Could you check a few things on this model? Use its own coordinates, in mm. A direction names the side the tool comes from. Give positions to 0.01 mm unless a question says otherwise; leave off trailing zeros. Write each loop counter-clockwise with the first axis right and the second up, starting at its lowest first coordinate (ties: lowest second). Pieces come first, ordered by that corner, then holes. Notation, with made-up numbers: M -23,46.5 L 18,46.5 A10 cw 18,62.5 Z; hole C -26,80.5 d2. An arc over 180 degrees is marked long. One line per item, written item: value.
```python
from build123d import *

# Parameters (mm, degrees)
SKETCH1_W           = 119.5324
SKETCH1_H           = 78.0034
BOSS_EXTRUDE1_DEPTH = 1.5875
CUT_EXTRUDE1_REACH  = 3.587
SKETCH2_R           = 2
SKETCH3_R           = 0.508
CUT_EXTRUDE2_DEPTH  = 1.5875
CUT_EXTRUDE4_REACH  = 3.587
LPATTERN1_COUNT     = 26
LPATTERN1_PITCH     = 2.54
SKETCH5_W           = 105.5
SKETCH5_H           = 67.2
BOSS_EXTRUDE2_DEPTH = 5.08
SKETCH6_W           = 98.5
SKETCH6_H           = 57.4
CUT_EXTRUDE3_DEPTH  = 0.127
SKETCH7_W           = 6
SKETCH7_H           = 3.5
BOSS_EXTRUDE3_DEPTH = 3.8
SKETCH8_W           = 3
SKETCH8_H           = 1.5
BOSS_EXTRUDE4_DEPTH = 0.7
SKETCH9_W           = 3
SKETCH9_H           = 3
BOSS_EXTRUDE5_DEPTH = 1.71
SKETCH10_W          = 3
SKETCH10_H          = 3
BOSS_EXTRUDE6_DEPTH = 1


with BuildPart() as part:
    # Sketch1 → Boss-Extrude1 (new body)
    with BuildSketch(Plane(origin=(0, 0, 0), x_dir=(1, 0, 0), z_dir=(0, 1, 0))):
        Rectangle(SKETCH1_W, SKETCH1_H)
    extrude(amount=BOSS_EXTRUDE1_DEPTH)

    # Sketch2 → Cut-Extrude1 (cut, up to next)
    with BuildSketch(Plane(origin=(0, 1.5875, 0), x_dir=(1, 0, 0), z_dir=(0, 1, 0)), mode=Mode.PRIVATE) as cut_extrude1_sk1:
        with Locations((-55.7657, 35.0012)):
            Circle(SKETCH2_R)
    cut_extrude1_tool1 = extrude(cut_extrude1_sk1.sketch, amount=-CUT_EXTRUDE1_REACH, mode=Mode.PRIVATE) & part.part
    add(cut_extrude1_tool1.solids().sort_by_distance((-55.7657, 1.5875, -35.0012))[0], mode=Mode.SUBTRACT)
    # Sketch2 → Cut-Extrude1 (cut, up to next)
    with BuildSketch(Plane(origin=(0, 1.5875, 0), x_dir=(1, 0, 0), z_dir=(0, 1, 0)), mode=Mode.PRIVATE) as cut_extrude1_sk2:
        with Locations((-55.7657, -35.0012)):
            Circle(SKETCH2_R)
    cut_extrude1_tool2 = extrude(cut_extrude1_sk2.sketch, amount=-CUT_EXTRUDE1_REACH, mode=Mode.PRIVATE) & part.part
    add(cut_extrude1_tool2.solids().sort_by_distance((-55.7657, 1.5875, 35.0012))[0], mode=Mode.SUBTRACT)
    # Sketch2 → Cut-Extrude1 (cut, up to next)
    with BuildSketch(Plane(origin=(0, 1.5875, 0), x_dir=(1, 0, 0), z_dir=(0, 1, 0)), mode=Mode.PRIVATE) as cut_extrude1_sk3:
        with Locations((55.7657, 35.0012)):
            Circle(SKETCH2_R)
    cut_extrude1_tool3 = extrude(cut_extrude1_sk3.sketch, amount=-CUT_EXTRUDE1_REACH, mode=Mode.PRIVATE) & part.part
    add(cut_extrude1_tool3.solids().sort_by_distance((55.7657, 1.5875, -35.0012))[0], mode=Mode.SUBTRACT)
    # Sketch2 → Cut-Extrude1 (cut, up to next)
    with BuildSketch(Plane(origin=(0, 1.5875, 0), x_dir=(1, 0, 0), z_dir=(0, 1, 0)), mode=Mode.PRIVATE) as cut_extrude1_sk4:
        with Locations((55.7657, -35.0012)):
            Circle(SKETCH2_R)
    cut_extrude1_tool4 = extrude(cut_extrude1_sk4.sketch, amount=-CUT_EXTRUDE1_REACH, mode=Mode.PRIVATE) & part.part
    add(cut_extrude1_tool4.solids().sort_by_distance((55.7657, 1.5875, 35.0012))[0], mode=Mode.SUBTRACT)

    # Sketch3 → Cut-Extrude2 (cut)
    with BuildSketch(Plane(origin=(0, 1.5875, 0), x_dir=(1, 0, 0), z_dir=(0, 1, 0))):
        with Locations((-31.7373, 36.758)):
            Circle(SKETCH3_R)
        with Locations((-31.7373, -36.758)):
            Circle(SKETCH3_R)
    cut_extrude2 = extrude(amount=-CUT_EXTRUDE2_DEPTH, mode=Mode.SUBTRACT)

    # Sketch11 → Cut-Extrude4 (cut, up to next)
    with BuildSketch(Plane(origin=(0, 1.5875, 0), x_dir=(1, 0, 0), z_dir=(0, 1, 0)), mode=Mode.PRIVATE) as cut_extrude4_sk1:
        with BuildLine():
            Line((-59.7662, 35.0012), (-59.7662, 39.0017))
            Line((-59.7662, 39.0017), (-55.7657, 39.0017))
            ThreePointArc((-55.7657, 39.0017), (-58.594480678, 37.829980678), (-59.7662, 35.0012))
        make_face()
    cut_extrude4_tool1 = extrude(cut_extrude4_sk1.sketch, amount=-CUT_EXTRUDE4_REACH, mode=Mode.PRIVATE) & part.part
    add(cut_extrude4_tool1.solids().sort_by_distance((-58.872617, 1.5875, -38.108117))[0], mode=Mode.SUBTRACT)
    # Sketch11 → Cut-Extrude4 (cut, up to next)
    with BuildSketch(Plane(origin=(0, 1.5875, 0), x_dir=(1, 0, 0), z_dir=(0, 1, 0)), mode=Mode.PRIVATE) as cut_extrude4_sk2:
        with BuildLine():
            Line((-59.7662, -39.0017), (-55.7657, -39.0017))
            ThreePointArc((-55.7657, -39.0017), (-58.594480678, -37.829980678), (-59.7662, -35.0012))
            Line((-59.7662, -35.0012), (-59.7662, -39.0017))
        make_face()
    cut_extrude4_tool2 = extrude(cut_extrude4_sk2.sketch, amount=-CUT_EXTRUDE4_REACH, mode=Mode.PRIVATE) & part.part
    add(cut_extrude4_tool2.solids().sort_by_distance((-58.872617, 1.5875, 38.108117))[0], mode=Mode.SUBTRACT)
    # Sketch11 → Cut-Extrude4 (cut, up to next)
    with BuildSketch(Plane(origin=(0, 1.5875, 0), x_dir=(1, 0, 0), z_dir=(0, 1, 0)), mode=Mode.PRIVATE) as cut_extrude4_sk3:
        with BuildLine():
            Line((59.7662, -35.0012), (59.7662, -39.0017))
            Line((59.7662, -39.0017), (55.7657, -39.0017))
            ThreePointArc((55.7657, -39.0017), (58.594480678, -37.829980678), (59.7662, -35.0012))
        make_face()
    cut_extrude4_tool3 = extrude(cut_extrude4_sk3.sketch, amount=-CUT_EXTRUDE4_REACH, mode=Mode.PRIVATE) & part.part
    add(cut_extrude4_tool3.solids().sort_by_distance((58.872617, 1.5875, 38.108117))[0], mode=Mode.SUBTRACT)
    # Sketch11 → Cut-Extrude4 (cut, up to next)
    with BuildSketch(Plane(origin=(0, 1.5875, 0), x_dir=(1, 0, 0), z_dir=(0, 1, 0)), mode=Mode.PRIVATE) as cut_extrude4_sk4:
        with BuildLine():
            Line((59.7662, 39.0017), (55.7657, 39.0017))
            ThreePointArc((55.7657, 39.0017), (58.594480678, 37.829980678), (59.7662, 35.0012))
            Line((59.7662, 35.0012), (59.7662, 39.0017))
        make_face()
    cut_extrude4_tool4 = extrude(cut_extrude4_sk4.sketch, amount=-CUT_EXTRUDE4_REACH, mode=Mode.PRIVATE) & part.part
    add(cut_extrude4_tool4.solids().sort_by_distance((58.872617, 1.5875, -38.108117))[0], mode=Mode.SUBTRACT)

    # LPattern1: Cut-Extrude2 ×26
    with Locations(*[(i * LPATTERN1_PITCH, 0, 0) for i in range(1, LPATTERN1_COUNT)]):
        add(cut_extrude2, mode=Mode.SUBTRACT)

    # Sketch5 → Boss-Extrude2 (add)
    with BuildSketch(Plane(origin=(0, 1.5875, 0), x_dir=(1, 0, 0), z_dir=(0, 1, 0))):
        with Locations((0.0838, 0.4017)):
            Rectangle(SKETCH5_W, SKETCH5_H)
    extrude(amount=BOSS_EXTRUDE2_DEPTH)

    # Sketch6 → Cut-Extrude3 (cut)
    with BuildSketch(Plane(origin=(0, 6.6675, 0), x_dir=(1, 0, 0), z_dir=(0, 1, 0))):
        with Locations((0.0838, 2.8017)):
            Rectangle(SKETCH6_W, SKETCH6_H)
    extrude(amount=-CUT_EXTRUDE3_DEPTH, mode=Mode.SUBTRACT)

    # Sketch7 → Boss-Extrude3 (add)
    with BuildSketch(Plane(origin=(0, 1.5875, 0), x_dir=(1, 0, 0), z_dir=(0, 1, 0))):
        with Locations((-42.2662, 36.2517)):
            Rectangle(SKETCH7_W, SKETCH7_H)
    extrude(amount=BOSS_EXTRUDE3_DEPTH)

    # Sketch8 → Boss-Extrude4 (add)
    with BuildSketch(Plane(origin=(0, 5.3875, 0), x_dir=(1, 0, 0), z_dir=(0, 1, 0))):
        with Locations((-42.2662, 36.2517)):
            Rectangle(SKETCH8_W, SKETCH8_H)
    extrude(amount=BOSS_EXTRUDE4_DEPTH)

    # Sketch9 → Boss-Extrude5 (add)
    with BuildSketch(Plane(origin=(0, 1.5875, 0), x_dir=(1, 0, 0), z_dir=(0, 1, 0))):
        with Locations((-56.3862, 9.9017)):
            Rectangle(SKETCH9_W, SKETCH9_H)
    extrude(amount=BOSS_EXTRUDE5_DEPTH)

    # Sketch10 → Boss-Extrude6 (add)
    with BuildSketch(Plane(origin=(0, 1.5875, 0), x_dir=(1, 0, 0), z_dir=(0, 1, 0))):
        with Locations((-56.0462, -12.2417)):
            Rectangle(SKETCH10_W, SKETCH10_H)
    extrude(amount=BOSS_EXTRUDE6_DEPTH)


solid = part.part
```
1) On a 3-axis mill with a long thin cutter (end or side, diameter ignored), from which of +Z, -Z, +X, -X, +Y, -Y can I reach the whole of each face in a straight line? I mean faces 5 (the face through (-39.266, 3, -36)), 6 (the face through (-1, 4, 33.198)), 7 (the face through (-42, 3, -38.002)), 8 (the face through (-42, 3, -34.502)), 9 (the face through (-56, 2.588, 12)). Say none if no direction works.
Outcome:
face 5: -Z, +X, +Y
face 6: +Z, +X, -X, +Y
face 7: -Z, +X, -X, +Y
face 8: +X, -X, +Y
face 9: +Z, -X, +Y
2) Please list where these lines run through material, in increasing order: L1, parallel to Y at x = 17, z = 22; L2, parallel to Z at x = 9.5, y = 6; L3, parallel to Z at x = -43, y = 5.5. Write a range as from..to.
Outcome:
L1: y = 0..6.54
L2: z = -34..33.2
L3: z = -37..-35.5, -34..33.2
3) We'd pull the mould along X, two halves only. Please class faces 1 (the face through (-53.858, 0.805, -35.602)), 2 (the face through (-45.266, 3, -36)), 3 (the face through (-56, 3.298, -10)), 4 (the face through (55.505, 0.805, -36.984)): pulls with the +X half, pulls with the -X half, needs draft (parallel to the pull), parting line crosses it, or undercut.
Outcome:
face 1: undercut
face 2: pulls with the -X half
face 3: needs draft
face 4: undercut
4) I'm going to push flat-ended pins straight in: pin 1 (1.5 mm diameter, centred on x = 10, y = 4.5, fed in from +Z); pin 2 (0.8 mm diameter, centred on x = 8.9, z = 36.76, fed in from -Y); pin 3 (1 mm diameter, centred on x = 26.5, y = 3, fed in from -Z); pin 4 (1.2 mm diameter, centred on x = 31.76, z = -36.76, fed in from +Y). Where does each tip first touch, or does it pass through?
Outcome:
pin 1: stops at z = 33.2
pin 2: passes through
pin 3: stops at z = -34
pin 4: stops at y = 1.59
5) If we section it at A-A, the plane z = 30.5: Write out the boundary of the cut face in (x, y).
Outcome:
outline: M -59.77,0 L 59.77,0 L 59.77,1.59 L 52.83,1.59 L 52.83,6.67 L -52.67,6.67 L -52.67,1.59 L -59.77,1.59 Z
6) If we section it at B-B, the plane x = 46: Write out the boundary of the cut face in (y, z), then the cut area to 3 significant figures.
Outcome:
outline: M 0,-39 L 1.59,-39 L 1.59,-34 L 6.67,-34 L 6.67,-31.5 L 6.54,-31.5 L 6.54,25.9 L 6.67,25.9 L 6.67,33.2 L 1.59,33.2 L 1.59,39 L 0,39 Z
area: 458 mm^2
